Can you work these out from the model? Positions are in its coordinate system, mm. Face numbers are marked on the shaded views. A direction names the side the tool comes from. Coordinates: 2 decimals unless noted, no trailing zeros. Loops run counter-clockwise (first coordinate to the right, second up) from the corner with the lowest first, then second, coordinate; pieces in that order, holes last.
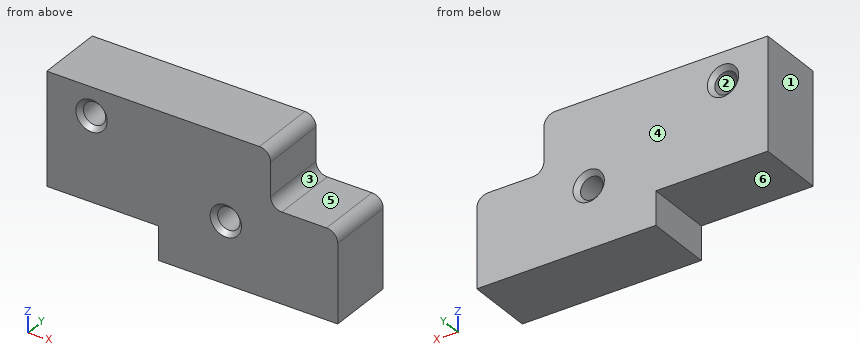
```python
from build123d import *

# Parameters (mm, degrees)
F1_DEPTH = 15
F2_R     = 5
F3_R     = 5
F4_DEPTH = 30.001
F5_SIZE  = 2


with BuildPart() as f1:
    # F0 (on Front) → F1 (new body, symmetric)
    with BuildSketch(Plane.XZ):
        Polygon((50, 25), (-50, 25), (-50, -25), (0, -25), (0, -40), (80, -40), (80, 0), (50, 0), align=None)
    extrude(amount=F1_DEPTH, both=True)

    # F2
    f2_edges = [f1.edges().sort_by_distance(p)[0] for p in [
        (50, 0, 0),
        (50, 0, 25),
        (80, 0, 0),
    ]]
    fillet(f2_edges, radius=F2_R)

    # F3 (on face) → F4 (cut, through all)
    with BuildSketch(Plane.XZ.offset(15)):
        with Locations((-30, 12.5)):
            Circle(F3_R)
        with Locations((30, -12.5)):
            Circle(F3_R)
    extrude(amount=-F4_DEPTH, mode=Mode.SUBTRACT)

    # F5
    f5_edges = [f1.edges().sort_by_distance(p)[0] for p in [
        (-35, -15, 12.5),
        (25, -15, -12.5),
        (-35, 15, 12.5),
        (25, 15, -12.5),
    ]]
    chamfer(f5_edges, length=F5_SIZE)


solid = f1.part
```
(1) If I drill on probe 1 along Z at (x, y) = (-30, -7); probe 2 along Z at (x, y) = (30, -5); probe 3 along X at (y, z) = (-3.75, 12), over which ranges is the centre line in solid material (lowest first)?
Check values:
probe 1: z = -25 to 7.5, 17.5 to 25
probe 2: z = -40 to -17.5, -7.5 to 25
probe 3: x = -50 to -34.97, -25.03 to 50
(2) I'm going to push flat-ended pins straight in: pin 1 (11.5 mm diameter, centred on x = 30, z = -12.5, fed in from -Y); pin 2 (10 mm diameter, centred on x = -9, z = -25.5, fed in from +Y); pin 3 (16.5 mm diameter, centred on y = -1, z = 15, fed in from +X); pin 4 (7.5 mm diameter, centred on y = -2.5, z = -33.5, fed in from -X). Where does each tip first touch, or does it pass through?
Check values:
pin 1: stops at y = -13.75
pin 2: stops at y = 15
pin 3: stops at x = 50
pin 4: stops at x = 0
(3) I want a section at C-C on x = -30. Write out the boundary of the cut face in (y, z).
Check values:
outline: (-15, -25) - (15, -25) - (15, 5.5) - (13, 7.5) - (-13, 7.5) - (-15, 5.5) - close; (-15, 19.5) - (-13, 17.5) - (13, 17.5) - (15, 19.5) - (15, 25) - (-15, 25) - close
(4) If we mould it in two halves opening along Z, with no side actions, what happens to the marked faces 1, 2 and 3? For each: released by +Z, released by -Z, zero draft, split by the parting line, or undercut.
Check values:
face 1: zero draft
face 2: undercut
face 3: released by +Z
(5) I want a section at D-D on z = 3. Write out the boundary of the cut face in (x, y).
Check values:
outline: (-50, -15) - (50.42, -15) - (50.42, 15) - (-50, 15) - close
(6) I want a section at B-B on y = 5.5. Write out the boundary of the cut face in (x, z).
Check values:
outline: (-50, -25) - (0, -25) - (0, -40) - (80, -40) - (80, -5) arc R5 ccw to (75, 0) - (55, 0) arc R5 cw to (50, 5) - (50, 20) arc R5 ccw to (45, 25) - (-50, 25) - close; hole circle Ø10 at (-30, 12.5); hole circle Ø10 at (30, -12.5)
(7) I want a section at A-A on z = 12.5. Write out the boundary of the cut face in (x, y).
Check values:
outline: (-50, -15) - (-37, -15) - (-35, -13) - (-35, 13) - (-37, 15) - (-50, 15) - close; (-25, -13) - (-23, -15) - (50, -15) - (50, 15) - (-23, 15) - (-25, 13) - close
(8) Which directions (+Z, -Z, +X, -X, +Y, -Y) give clear straight access to the entire face, cutting with the end or side of a thin tool? Please do the marked faces 4, 5 and 6.
Check values:
face 4: +Z, -Z, +X, -X, +Y
face 5: +Z, +X, +Y, -Y
face 6: -Z, -X, +Y, -Y
